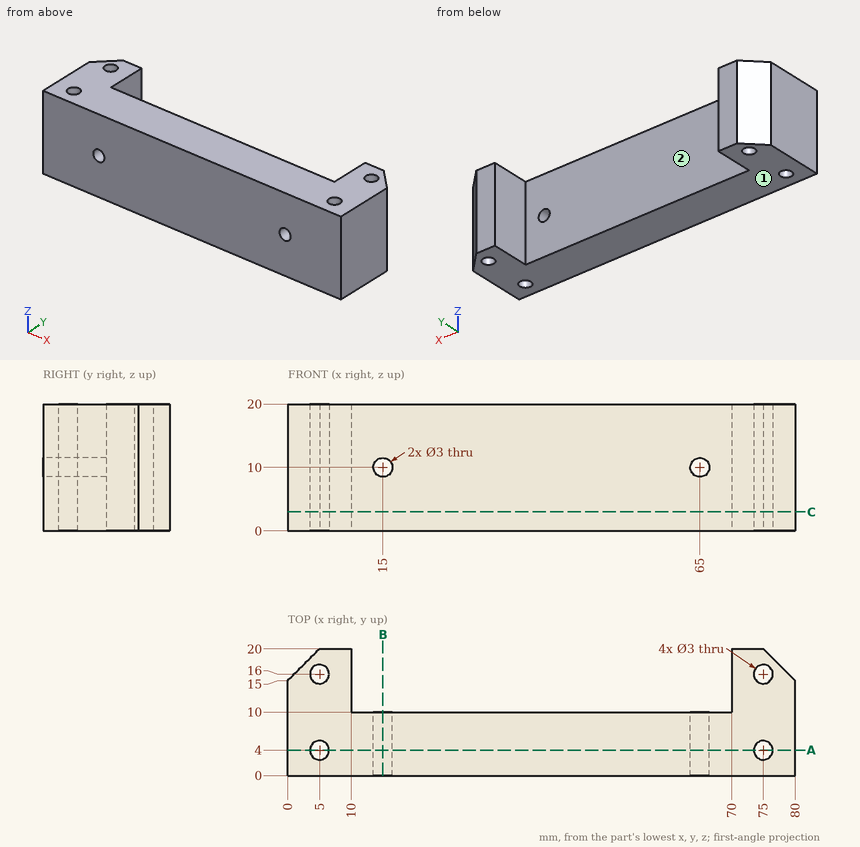
Answer from the drawing. Dimensions are ordinates in mm from the lowest x, y and z of the part. A direction names the side the tool comes from. Round coordinates to 2 decimals unless told otherwise and drop trailing zeros. Loops run counter-clockwise (first coordinate to the right, second up) from the corner with the lowest first, then second, coordinate; pieces in that order, holes last.
Q1. Consider probe 1 along Y at (x, z) = (75, 13.5); probe 2 along X at (y, z) = (11.75, 4.25); probe 3 along Y at (x, z) = (76, 11). Determine where each line is inside the solid, lowest interval first.
Q2. Section C-C on z = 3 is taken. Write down the section's boundary in (x, y), and give its area (3 significant figures).
Q3. Which of the six approach directions +Z, -Z, +X, -X, +Y, -Y give full straight-line access (tool end or side, diameter ignored) to the marked faces 1 and 2?
Q4. Each of these flat-tipped pins is pushed along its axis until it touches: pin 1 (4 mm diameter, centred on x = 5, y = 4, fed in from +Z); pin 2 (2.5 mm diameter, centred on x = 75, y = 16, fed in from +Z); pin 3 (2 mm diameter, centred on x = 57.5, z = 4.5, fed in from +Y); pin 4 (3 mm diameter, centred on y = 17, z = 9, fed in from +X). Where does it stop, or does it pass through?
Q5. Section B-B on x = 15 is taken. Write down the section's boundary in (y, z), and give its area (3 significant figures).
Q6. Section A-A on y = 4 is taken. Write down the section's boundary in (x, z), and give its area (3 significant figures).
Output:
1. probe 1: y = 0 to 2.5, 5.5 to 14.5, 17.5 to 20
1. probe 2: x = 0 to 10, 70 to 80
1. probe 3: y = 0 to 2.88, 5.12 to 14.88, 17.12 to 19
2. outline: (0, 0) - (80, 0) - (80, 15) - (75, 20) - (70, 20) - (70, 10) - (10, 10) - (10, 20) - (5, 20) - (0, 15) - close; hole circle Ø3 at (5, 4); hole circle Ø3 at (5, 16); hole circle Ø3 at (75, 4); hole circle Ø3 at (75, 16)
2. area: 947 mm2
3. face 1: -Z, +X, -X, +Y, -Y
3. face 2: +Z, -Z, +Y
4. pin 1: stops at z = 20
4. pin 2: passes through
4. pin 3: stops at y = 10
4. pin 4: stops at x = 79.5
5. outline: (0, 0) - (10, 0) - (10, 8.5) - (0, 8.5) - close; (0, 11.5) - (10, 11.5) - (10, 20) - (0, 20) - close
5. area: 170 mm2
6. outline: (0, 0) - (3.5, 0) - (3.5, 20) - (0, 20) - close; (6.5, 0) - (73.5, 0) - (73.5, 20) - (6.5, 20) - close; (76.5, 0) - (80, 0) - (80, 20) - (76.5, 20) - close; hole circle Ø3 at (15, 10); hole circle Ø3 at (65, 10)
6. area: 1,470 mm2
